Here's how the part is built. I have some questions about the finished solid (model axes, mm). A direction names the side the tool comes from. Give positions to 0.01 mm unless a question says otherwise; leave off trailing zeros. Loops run counter-clockwise (first coordinate to the right, second up) from the corner with the lowest first, then second, coordinate; pieces in that order, holes last.
Q1. I'm going to push flat-ended pins straight in: P1, Ø12, axis at x = -14, y = 1, coming from the -Z side; P2, Ø3, axis at x = 1, y = -4, coming from the +Z side; P3, Ø0.5, axis at x = -18, z = 3.5, coming from the +Y side. Where does each tip first touch, or does it pass through?
Q2. Suppose I cut it at D-D (z = 2). List the corners of the cut face in (x, y) for me.
Q3. For faces 4 (the face through (-34.341, 0, 6)), 5 (the face through (26.541, -13.016, -0.493)), 6 (the face through (-38.341, 0, 4)), 7 (the face through (34, 4.879, 7)), 8 (the face through (-4.341, 18, 6)), which set-ups out of +Z, -Z, +X, -X, +Y, -Y let a thin tool reach every point of the face, with its end or its side?
Q4. Suppose I cut it at A-A (y = 3). List the corners of the cut face in (x, z) for me, and give its area (3 significant figures).
Q5. Suppose I cut it at B-B (z = 5). List the corners of the cut face in (x, y) for me.
Q6. Thinking about a two-plate mould opening in Y: for faces 1 (the face through (-1, 20.079, 3)), 2 (the face through (34, -6.121, 7)), 3 (the face through (28, 12, -1)), which applies, pulls with the +Y half, pulls with the -Y half, needs draft (parallel to the pull), parting line crosses it, or undercut?
Q7. Suppose I cut it at C-C (x = 15). List the corners of the cut face in (y, z) for me, and give its area (3 significant figures).
Q8. I need wall thicknesses on probe 1 along Y at (x, z) = (-2, 4.25); probe 2 along X at (y, z) = (-8.5, 4.25); probe 3 along Y at (x, z) = (9.5, 0.25). Which ranges of each line are inside material? Lowest first, please.
```python
from build123d import *

# Parameters (mm, degrees)
SKETCH_1_W          = 74.8
SKETCH_1_H          = 40.3
EXTRUDE_1_DEPTH     = 4
SKETCH_2_W          = 74.8
SKETCH_2_H          = 40.3
SKETCH_2_W_2        = 66.8
SKETCH_2_H_2        = 32.3
EXTRUDE_1_2_DEPTH   = 4
SKETCH_3_R          = 2.125481821
SKETCH_3_R_2        = 2.41676927
SKETCH_3_R_3        = 2.07603791
SKETCH_3_R_4        = 2.373619113
EXTRUDE_2_DEPTH     = 1
SKETCH_4_W          = 4
SKETCH_4_H          = 11
CUT_EXTRUDE_1_DEPTH = 2
SKETCH_6_W          = 66.8
SKETCH_6_H          = 8.5
CUT_EXTRUDE_3_DEPTH = 1.2
SKETCH_7_W          = 13
SKETCH_7_H          = 4
SKETCH_7_W_2        = 22.6
CUT_EXTRUDE_4_DEPTH = 5
CUT_EXTRUDE_5_REACH = 7
SKETCH_9_W          = 12.4
SKETCH_9_H          = 12.4


with BuildPart() as part:
    # 草圖1 → Extrude 1 (new body)
    with BuildSketch(Plane.XY):
        with Locations((-0.94084879, -0.070758559)):
            Rectangle(SKETCH_1_W, SKETCH_1_H)
    extrude(amount=EXTRUDE_1_DEPTH)

    # 草圖2 → Extrude 1 2 (add)
    with BuildSketch(Plane.XY.offset(4)):
        with Locations((-0.94084879, -0.070758559)):
            Rectangle(SKETCH_2_W, SKETCH_2_H)
        with Locations((-0.94084879, -0.070758559)):
            Rectangle(SKETCH_2_W_2, SKETCH_2_H_2, mode=Mode.SUBTRACT)
    extrude(amount=EXTRUDE_1_2_DEPTH)

    # 草圖3 → 填料-伸長2 (add)
    with BuildSketch(Plane(origin=(0, 0, 0), x_dir=(-1, 0, 0), z_dir=(0, 0, -1))):
        with Locations((-28.45915121, 12.079241441)):
            Circle(SKETCH_3_R)
        with Locations((30.34084879, 12.079241441)):
            Circle(SKETCH_3_R_2)
        with Locations((-28.45915121, -12.220758559)):
            Circle(SKETCH_3_R_3)
        with Locations((30.34084879, -12.220758559)):
            Circle(SKETCH_3_R_4)
    extrude(amount=EXTRUDE_2_DEPTH)

    # 草圖4 → 除料-伸長1 (cut)
    with BuildSketch(Plane.XY.offset(8)):
        with Locations((34.45915121, -0.620758559)):
            Rectangle(SKETCH_4_W, SKETCH_4_H)
    extrude(amount=-CUT_EXTRUDE_1_DEPTH, mode=Mode.SUBTRACT)

    # 草圖6 → 除料-伸長3 (cut)
    with BuildSketch(Plane.XY.offset(4)):
        with Locations((-0.94084879, -11.970758559)):
            Rectangle(SKETCH_6_W, SKETCH_6_H)
    extrude(amount=-CUT_EXTRUDE_3_DEPTH, mode=Mode.SUBTRACT)

    # 草圖7 → 除料-伸長4 (cut)
    with BuildSketch(Plane.XY.offset(8)):
        with Locations((19.95915121, 18.079241441)):
            Rectangle(SKETCH_7_W, SKETCH_7_H)
        with Locations((-15.64084879, 18.079241441)):
            Rectangle(SKETCH_7_W_2, SKETCH_7_H)
    extrude(amount=-CUT_EXTRUDE_4_DEPTH, mode=Mode.SUBTRACT)

    # 草圖9 → 除料-伸長5 (cut, up to next)
    with BuildSketch(Plane.XY.offset(4), mode=Mode.PRIVATE) as cut_extrude_5_sk1:
        with Locations((6.65915121, 1.279241441)):
            Rectangle(SKETCH_9_W, SKETCH_9_H)
    cut_extrude_5_tool1 = extrude(cut_extrude_5_sk1.sketch, amount=-CUT_EXTRUDE_5_REACH, mode=Mode.PRIVATE) & part.part
    add(cut_extrude_5_tool1.solids().sort_by_distance((6.659151, 1.279241, 4))[0], mode=Mode.SUBTRACT)


solid = part.part
```
Solutions:
1. P1: stops at z = 0
1. P2: stops at z = 4
1. P3: stops at y = 16.08
2. outline: (-38.34, -20.22) - (36.46, -20.22) - (36.46, 20.08) - (-38.34, 20.08) - close; hole (0.46, -4.92) - (12.86, -4.92) - (12.86, 7.48) - (0.46, 7.48) - close
3. face 4: +Z
3. face 5: -Z
3. face 6: +Z, -Z, -X, +Y, -Y
3. face 7: +Z, +X
3. face 8: +Z, +Y
4. outline: (-38.34, 0) - (0.46, 0) - (0.46, 4) - (-34.34, 4) - (-34.34, 8) - (-38.34, 8) - close; (12.86, 0) - (36.46, 0) - (36.46, 6) - (32.46, 6) - (32.46, 4) - (12.86, 4) - close
4. area: 274 mm2
5. outline: (-38.34, -20.22) - (36.46, -20.22) - (36.46, 20.08) - (26.46, 20.08) - (26.46, 16.08) - (32.46, 16.08) - (32.46, -16.22) - (-34.34, -16.22) - (-34.34, 16.08) - (-26.94, 16.08) - (-26.94, 20.08) - (-38.34, 20.08) - close; (-4.34, 16.08) - (13.46, 16.08) - (13.46, 20.08) - (-4.34, 20.08) - close
6. face 1: pulls with the +Y half
6. face 2: undercut
6. face 3: needs draft
7. outline: (-20.22, 0) - (20.08, 0) - (20.08, 3) - (16.08, 3) - (16.08, 4) - (-7.72, 4) - (-7.72, 2.8) - (-16.22, 2.8) - (-16.22, 8) - (-20.22, 8) - close
7. area: 163 mm2
8. probe 1: y = -20.22 to -16.22, 16.08 to 20.08
8. probe 2: x = -38.34 to -34.34, 32.46 to 36.46
8. probe 3: y = -20.22 to -4.92, 7.48 to 20.08
